```python
from build123d import *

# Parameters (mm, degrees)
SKETCH_1_W          = 19.8
SKETCH_1_H          = 10.4
EXTRUDE_1_DEPTH     = 6.4
SKETCH_2_R          = 1.3
CUT_EXTRUDE_1_DEPTH = 13.884486796
EXTRUDE_2_DEPTH     = 0.8
EXTRUDE_3_DEPTH     = 0.8
EXTRUDE_4_DEPTH     = 0.8
SKETCH_8_R          = 0.8
CUT_EXTRUDE_3_DEPTH = 22.33096341
CUT_EXTRUDE_4_DEPTH = 15.892279879
FILLET_3_R          = 1
EXTRUDE_5_DEPTH     = 4
EXTRUDE_10_DEPTH    = 4
FILLET_4_R          = 0.5
FILLET_5_R          = 1
FILLET_6_R          = 1
FILLET_7_R          = 1
EXTRUDE_11_DEPTH    = 6.4


with BuildPart() as part:
    # 草图1 → 凸台-拉伸1 (new body)
    with BuildSketch(Plane.XY):
        Rectangle(SKETCH_1_W, SKETCH_1_H)
    extrude(amount=EXTRUDE_1_DEPTH)

    # 草图2 → 切除-拉伸1 (cut, through all)
    with BuildSketch(Plane(origin=(0, 0, 0), x_dir=(-1, 0, 0), z_dir=(0, 0, -1))):
        with Locations((-4.75, -2.8)):
            Circle(SKETCH_2_R)
        with Locations((4.75, -2.8)):
            Circle(SKETCH_2_R)
    extrude(amount=-CUT_EXTRUDE_1_DEPTH, mode=Mode.SUBTRACT)

    # 草图5 → 凸台-拉伸2 (add)
    with BuildSketch(Plane(origin=(8.3, 0, 0), x_dir=(0, 0, -1), z_dir=(1, 0, 0))):
        with BuildLine():
            Line((-4.8, -5.2), (-1.6, -5.2))
            Line((-1.6, -5.2), (-1.6, -8.6))
            ThreePointArc((-1.6, -8.6), (-1.746446609, -8.953553391), (-2.1, -9.1))
            Line((-2.1, -9.1), (-4.3, -9.1))
            ThreePointArc((-4.3, -9.1), (-4.653553391, -8.953553391), (-4.8, -8.6))
            Line((-4.8, -8.6), (-4.8, -5.2))
        make_face()
    extrude(amount=-EXTRUDE_2_DEPTH)

    # 草图6 → 凸台-拉伸3 (add)
    with BuildSketch(Plane(origin=(-0.5, 0, 0), x_dir=(0, 0, -1), z_dir=(1, 0, 0))):
        with BuildLine():
            Line((-4.8, -5.2), (-1.6, -5.2))
            Line((-1.6, -5.2), (-1.6, -8.6))
            ThreePointArc((-1.6, -8.6), (-1.746446609, -8.953553391), (-2.1, -9.1))
            Line((-2.1, -9.1), (-4.3, -9.1))
            ThreePointArc((-4.3, -9.1), (-4.653553391, -8.953553391), (-4.8, -8.6))
            Line((-4.8, -8.6), (-4.8, -5.2))
        make_face()
    extrude(amount=-EXTRUDE_3_DEPTH)

    # 草图7 → 凸台-拉伸4 (add)
    with BuildSketch(Plane(origin=(-7.8, 0, 0), x_dir=(0, 0, -1), z_dir=(1, 0, 0))):
        with BuildLine():
            Line((-4.8, -5.2), (-1.6, -5.2))
            Line((-1.6, -5.2), (-1.6, -8.6))
            ThreePointArc((-1.6, -8.6), (-1.746446609, -8.953553391), (-2.1, -9.1))
            Line((-2.1, -9.1), (-4.3, -9.1))
            ThreePointArc((-4.3, -9.1), (-4.653553391, -8.953553391), (-4.8, -8.6))
            Line((-4.8, -8.6), (-4.8, -5.2))
        make_face()
    extrude(amount=-EXTRUDE_4_DEPTH)

    # 草图8 → 切除-拉伸3 (cut, through all)
    with BuildSketch(Plane(origin=(8.3, 0, 0), x_dir=(0, 0, -1), z_dir=(1, 0, 0))):
        with Locations(Location((-3.2, -7.6, 0), (0, 0, 180))):
            Circle(SKETCH_8_R)
    extrude(amount=-CUT_EXTRUDE_3_DEPTH, mode=Mode.SUBTRACT)

    # 草图9 → 切除-拉伸4 (cut, through all)
    with BuildSketch(Plane(origin=(0, 0, 0), x_dir=(-1, 0, 0), z_dir=(0, 0, -1))):
        Polygon((-1.9, 5.2), (-0.6, 4.4), (9.9, 4.4), (9.9, 5.2), align=None)
    extrude(amount=-CUT_EXTRUDE_4_DEPTH, mode=Mode.SUBTRACT)

    # 圆角3
    fillet_3_edges = [part.edges().sort_by_distance(p)[0] for p in [
        (1.9, 5.2, 3.2),
        (0.6, 4.4, 3.2),
    ]]
    fillet(fillet_3_edges, radius=FILLET_3_R)

    # 草图10 → 凸台-拉伸5 (add)
    with BuildSketch(Plane.XY.offset(1.2)):
        with BuildLine():
            Line((3.15, 5.2), (4.65, 5.2))
            Line((4.65, 5.2), (4.65, 5.3))
            ThreePointArc((4.65, 5.3), (3.9, 6.05), (3.15, 5.3))
            Line((3.15, 5.3), (3.15, 5.2))
        make_face()
    extrude(amount=EXTRUDE_5_DEPTH)

    # 草图12 → 凸台-拉伸10 (add)
    with BuildSketch(Plane.XY.offset(1.2)):
        Polygon((7.4, 5.2), (7.4, 5), (7.7, 5), (7.7, 5.2), (7.7, 5.965506001), (-9.713537643, 8.097775917), (-9.75, 7.8), (7.4, 5.7), align=None)
    extrude(amount=EXTRUDE_10_DEPTH)

    # 圆角4
    fillet_4_edges = [part.edges().sort_by_distance(p)[0] for p in [
        (7.4, 5.7, 3.2),
    ]]
    fillet(fillet_4_edges, radius=FILLET_4_R)

    # 圆角5
    # the kernel refuses this fillet: 1 mm, written as the material it takes off along each edge
    with BuildSketch(Plane(origin=(7.7, 5.965506001, -0.994226351), x_dir=(0, -1, 0), z_dir=(0, 0, 1))) as fillet_5_piece_1:
        with BuildLine():
            CenterArc((0.885910836, -0.992724874), FILLET_5_R, 96.915467292, 76.103475301)
            Line((-0.106675553, -0.871183684), (-0.126527281, -0.86875286))
            Line((-0.126527281, -0.86875286), (-0.019851728, 0.002430824))
            Line((-0.019851728, 0.002430824), (0, 0.02))
            ThreePointArc((0, 0.02), (0.382753001, 0.02), (0.763097904, 0.019854497))
            Line((0.763097904, 0.019854497), (0.765506001, 0))
        make_face()
    extrude(amount=8.388452701, mode=Mode.SUBTRACT)

    # 圆角6
    fillet_6_edges = [part.edges().sort_by_distance(p)[0] for p in [
        (9.9, -5.2, 3.2),
        (-9.9, -5.2, 3.2),
    ]]
    fillet(fillet_6_edges, radius=FILLET_6_R)

    # 圆角7
    fillet_7_edges = [part.edges().sort_by_distance(p)[0] for p in [
        (9.9, 5.2, 3.2),
        (-9.9, 4.4, 3.2),
    ]]
    fillet(fillet_7_edges, radius=FILLET_7_R)

    # 草图13 → 凸台-拉伸11 (add)
    with BuildSketch(Plane.XY.offset(6.4)):
        Polygon((-6.55, -5.2), (-6.25, -5.6), (-3.25, -5.6), (-2.95, -5.2), align=None)
        Polygon((6.25, -5.6), (3.25, -5.6), (2.95, -5.2), (6.55, -5.2), align=None)
    extrude(amount=-EXTRUDE_11_DEPTH)


solid = part.part
```
Check sheet for the modelled part. Datum: model origin and axes. Units: mm. A direction names the side the tool comes from. Round coordinates to 2 decimals unless told otherwise and drop trailing zeros. Loops run counter-clockwise (first coordinate to the right, second up) from the corner with the lowest first, then second, coordinate; pieces in that order, holes last. Notation, with made-up numbers: (-2, 21.25) -> (44, 21.25) arc R13 cw to (44, 26.25) -> close; hole circle Ø4 at (-11, 40.5). An arc over 180 degrees is marked (long way). Write item = value, one per line. Start each with the question number.
1) Sectioned sample at B-B, the plane x = -4. Record the cut outline in (y, z), plus the area to 3 significant figures.
2) Thickness scan on probe 1 along Z at (x, y) = (-0.9, -7.6); probe 2 along Y at (x, z) = (4.75, 4); probe 3 along Y at (x, z) = (-1.1, 3.2). Record the ranges inside material, lowest first.
3) Sectioned sample at A-A, the plane y = -2.8. Record the cut outline in (x, z), plus the area to 3 significant figures.
4) Set-up check for faces 1 (the flat face through (8.3, -6.7, 2.8)), 2 (the cylindrical face through (-8.19, -6.82, 3.03)), 3 (the flat face through (3.9, 5.5, 1.2)), 4 (the flat face through (-7.8, -6.7, 2.8)), 5 (the flat face through (-4, 4.4, 3)): record each of +Z, -Z, +X, -X, +Y, -Y from which the full face is reachable in a straight line by a thin tool's end or side.
5) Sectioned sample at C-C, the plane z = 3.2. State how many separate pieces and enclosed holes the cut face has, plus the area to 3 significant figures.
6) Gauge pin test, flat ends, axial feed: pin 1 Ø1.8 at (y, z) = (-7.6, 3.2) entering from +X; pin 2 Ø1 at (x, z) = (-6.5, 4) entering from -Y; pin 3 Ø2 at (x, z) = (3.5, 3.5) entering from +Y. Record the tip position at first contact, or that the pin passes through.
7) Release check for a two-part mould opening along X. For faces 6 (the cylindrical face through (-5.99, -2.41, 3.16)), 7 (the flat face through (3.9, 5.5, 5.2)), 8 (the flat face through (-0.5, -6.7, 2.8)), 9 (the cylindrical face through (9.599, -4.915, 3.245)) record: released by +X, released by -X, zero draft, split by the parting line, or undercut.
8) Sectioned sample at D-D, the plane x = 2.5. Record the cut outline in (y, z).
Results are:
q1.outline = (-5.6, 0) -> (-3.86, 0) -> (-3.86, 6.4) -> (-5.6, 6.4) -> close; (-1.74, 0) -> (4.4, 0) -> (4.4, 6.4) -> (-1.74, 6.4) -> close; (7.1, 1.2) -> (7.4, 1.2) -> (7.4, 5.2) -> (7.1, 5.2) -> close
q1.area = 51.6 mm^2
q2.probe_1 = 1.6 to 2.4, 4 to 4.8
q2.probe_2 = -5.6 to -4.1, -1.5 to 5.2, 6.02 to 6.33
q2.probe_3 = -9.1 to -8.4, -6.8 to 4.4, 6.74 to 7.04
q3.outline = (-9.9, 0) -> (-6.05, 0) -> (-6.05, 6.4) -> (-9.9, 6.4) -> close; (-3.45, 0) -> (3.45, 0) -> (3.45, 6.4) -> (-3.45, 6.4) -> close; (6.05, 0) -> (9.9, 0) -> (9.9, 6.4) -> (6.05, 6.4) -> close
q3.area = 93.4 mm^2
q4.face_1 = +Z, -Z, +X, -Y
q4.face_2 = +X, -X
q4.face_3 = -Z, +X, -X, +Y
q4.face_4 = +Z, -Z, -Y
q4.face_5 = +Z, -Z, -X
q5.separate_pieces = 4
q5.enclosed_holes = 2
q5.area = 200 mm^2
q6.pin_1 = 8.3
q6.pin_2 = -5.6
q6.pin_3 = 6.6
q7.face_6 = undercut
q7.face_7 = zero draft
q7.face_8 = undercut
q7.face_9 = released by +X
q8.outline = (-5.2, 0) -> (5.2, 0) -> (5.2, 6.4) -> (-5.2, 6.4) -> close; (6.3, 1.2) -> (6.6, 1.2) -> (6.6, 5.2) -> (6.3, 5.2) -> close
